Source: CAD feature listing. Evaluate the final solid. Frame: model axes, mm. Coordinates: 2 decimals unless noted, no trailing zeros. Order: outer loops, then holes, each group sorted by start corner. A loop starts at its lowest first (then second) coordinate and runs counter-clockwise, first axis right, second up. Notation, with made-up numbers: (85, 43.25) -> (116, 43.25) arc R23 cw to (116, 82.25) -> close; hole circle Ø2 at (-10, 12.25). An arc over 180 degrees is marked (long way). Put each result on its own line as item: value.
from build123d import *

# Parameters (mm, degrees)
SZKIC1_R                    = 10
DODANIE_WYCI_GNI_CIE1_DEPTH = 5
SZKIC2_OUTSIDE_W            = 76.022
SZKIC2_OUTSIDE_H            = 80.664
SZKIC2_OUTSIDE_R            = 15
WYTNIJ_WYCI_GNI_CIE2_DEPTH  = 10
WYTNIJ_WYCI_GNI_CIE2_DRAFT  = -60
LUSTRO1_COPY_1_SKETCH_W     = 76.022
LUSTRO1_COPY_1_SKETCH_H     = 80.664
LUSTRO1_COPY_1_SKETCH_R     = 15
LUSTRO1_COPY_1_DEPTH        = 10
LUSTRO1_COPY_1_DRAFT        = -60


with BuildPart() as part:
    # Szkic1 → Dodanie-wyciągnięcie1 (new, symmetric)
    with BuildSketch(Plane.XY):
        Polygon((-15, 8.660254038), (-15, -8.660254038), (0, -17.320508076), (15, -8.660254038), (15, 8.660254038), (0, 17.320508076), align=None)
        Circle(SZKIC1_R, mode=Mode.SUBTRACT)
    extrude(amount=DODANIE_WYCI_GNI_CIE1_DEPTH, both=True)


with BuildPart() as wytnij_wyci_gni_cie2_tool:
    # Szkic2 outside → Wytnij-wyciągnięcie2 (with draft: the straight prism first)
    with BuildSketch(Plane.XY.offset(5)):
        Rectangle(SZKIC2_OUTSIDE_W, SZKIC2_OUTSIDE_H)
        Circle(SZKIC2_OUTSIDE_R, mode=Mode.SUBTRACT)
    extrude(amount=-WYTNIJ_WYCI_GNI_CIE2_DEPTH)
    # Wytnij-wyciągnięcie2: the draft: its side faces are tilted about the plane it starts from
    wytnij_wyci_gni_cie2_sides = [wytnij_wyci_gni_cie2_tool.faces().sort_by_distance(p)[0] for p in [
        (0, -40.332, 0),
        (38.011, 0, 0),
        (0, 40.332, 0),
        (-38.011, 0, 0),
        (-15, 0, 0),
    ]]
    draft(wytnij_wyci_gni_cie2_sides, Plane.XY.offset(5), WYTNIJ_WYCI_GNI_CIE2_DRAFT)


with BuildPart() as part_1:
    add(part.part)

    # Wytnij-wyciągnięcie2: cut by wytnij_wyci_gni_cie2_tool
    add(wytnij_wyci_gni_cie2_tool.part, mode=Mode.SUBTRACT)


with BuildPart() as lustro1_copy_1_tool:
    # Lustro1 copy 1 sketch → Lustro1 copy 1 (with draft: the straight prism first)
    with BuildSketch(Plane(origin=(0, 0, -5), x_dir=(1, 0, 0), z_dir=(0, 0, -1))):
        Rectangle(LUSTRO1_COPY_1_SKETCH_W, LUSTRO1_COPY_1_SKETCH_H)
        Circle(LUSTRO1_COPY_1_SKETCH_R, mode=Mode.SUBTRACT)
    extrude(amount=-LUSTRO1_COPY_1_DEPTH)
    # Lustro1 copy 1: the draft: its side faces are tilted about the plane it starts from
    lustro1_copy_1_sides = [lustro1_copy_1_tool.faces().sort_by_distance(p)[0] for p in [
        (0, -40.332, 0),
        (38.011, 0, 0),
        (0, 40.332, 0),
        (-38.011, 0, 0),
        (-15, 0, 0),
    ]]
    draft(lustro1_copy_1_sides, Plane(origin=(0, 0, -5), x_dir=(1, 0, 0), z_dir=(0, 0, -1)), LUSTRO1_COPY_1_DRAFT)


with BuildPart() as part_2:
    add(part_1.part)

    # Lustro1 copy 1: cut by lustro1_copy_1_tool
    add(lustro1_copy_1_tool.part, mode=Mode.SUBTRACT)


solid = part_2.part
1. Cut plane A-A on z = -1.75. Output: boundary loops of the cut face in (x, y).
Numbers:
outline: (-15, -8.66) -> (0, -17.32) -> (15, -8.66) -> (15, 8.66) -> (0, 17.32) -> (-15, 8.66) -> close; hole circle Ø20 at (0, 0)
2. Ray query, line 1 along Y through (x, z) = (0, 2); line 2 along X through (y, z) = (-9, 0.25); line 3 along Y through (x, z) = (0, 3.75). Return the intervals inside material, ascending.
Numbers:
line 1: y = -17.32 to -10, 10 to 17.32
line 2: x = -14.41 to -4.36, 4.36 to 14.41
line 3: y = -17.17 to -10, 10 to 17.17
3. Pull-direction query (Y, two-part tool) for faces 1 (the flat face through (-15, 0, 0)), 2 (the cylindrical face through (-2.17, -9.76, -0.07)), 3 (the conical face through (13.49, 7.74, 4.68)); classes: pulls with the +Y half, pulls with the -Y half, needs draft (parallel to the pull), parting line crosses it, or undercut.
Numbers:
face 1: needs draft
face 2: undercut
face 3: pulls with the +Y half
4. First-contact query: pin 1 (1 mm diameter, centred on x = -5, z = 0, fed in from -Y); pin 2 (2 mm diameter, centred on y = 10, z = -1, fed in from -X); pin 3 (6 mm diameter, centred on y = 13.5, z = -2, fed in from -X); pin 4 (18 mm diameter, centred on x = 0, y = 0, fed in from -Z). Flat tips, straight axial feed; report the tip coordinate or a pass-through.
Numbers:
pin 1: stops at y = -14.72
pin 2: stops at x = -14.41
pin 3: stops at x = -11.81
pin 4: passes through
